```python
from build123d import *

# Parameters (mm, degrees)
CROQUIS1_R              = 1.75
SALIENTE_EXTRUIR1_DEPTH = 2
CROQUIS2_W              = 6
CROQUIS2_H              = 2
CORTAR_EXTRUIR1_DEPTH   = 1.2


with BuildPart() as part:
    # Croquis1 → Saliente-Extruir1 (new body)
    with BuildSketch(Plane(origin=(0, 0, 0), x_dir=(1, 0, 0), z_dir=(0, 1, 0))):
        with BuildLine():
            Line((-20.25, 0), (-20.25, 21))
            Line((-20.25, 21), (20.25, 21))
            Line((20.25, 21), (20.25, 0))
            Line((20.25, 0), (21.3, 0))
            Line((21.3, 0), (21.3, -3))
            Line((21.3, -3), (24.8, -3))
            Line((24.8, -3), (24.8, 0))
            Line((24.8, 0), (28.8, 0))
            Line((28.8, 0), (28.8, 18))
            ThreePointArc((28.8, 18), (27.335533906, 21.535533906), (23.8, 23))
            Line((23.8, 23), (-23.8, 23))
            ThreePointArc((-23.8, 23), (-27.335533906, 21.535533906), (-28.8, 18))
            Line((-28.8, 18), (-28.8, 0))
            Line((-28.8, 0), (-24.8, 0))
            Line((-24.8, 0), (-24.8, -3))
            Line((-24.8, -3), (-21.3, -3))
            Line((-21.3, -3), (-21.3, 0))
            Line((-21.3, 0), (-20.25, 0))
        make_face()
        with Locations(Location((-25, 5, 0), (0, 0, 270))):
            Circle(CROQUIS1_R, mode=Mode.SUBTRACT)
        with Locations(Location((25, 5, 0), (0, 0, 270))):
            Circle(CROQUIS1_R, mode=Mode.SUBTRACT)
        with Locations(Location((25, 16, 0), (0, 0, 270))):
            Circle(CROQUIS1_R, mode=Mode.SUBTRACT)
        with Locations(Location((-25, 16, 0), (0, 0, 270))):
            Circle(CROQUIS1_R, mode=Mode.SUBTRACT)
    extrude(amount=SALIENTE_EXTRUIR1_DEPTH)

    # Croquis2 → Cortar-Extruir1 (cut)
    with BuildSketch(Plane(origin=(0, 2, 0), x_dir=(1, 0, 0), z_dir=(0, 1, 0))):
        with Locations((-23.25, 10.5)):
            Rectangle(CROQUIS2_W, CROQUIS2_H)
        with Locations((23.25, 10.5)):
            Rectangle(CROQUIS2_W, CROQUIS2_H)
    extrude(amount=-CORTAR_EXTRUIR1_DEPTH, mode=Mode.SUBTRACT)


solid = part.part
```
CAD build for the part. Positions are in the model's coordinates, mm. A direction names the side the tool comes from. Coordinates: 2 decimals unless noted, no trailing zeros. Loops run counter-clockwise (first coordinate to the right, second up) from the corner with the lowest first, then second, coordinate; pieces in that order, holes last. Notation, with made-up numbers: (19.5, 71.25) - (27.5, 71.25) arc R27 cw to (27.5, 91.25) - close; hole circle Ø10 at (52, -11.5). An arc over 180 degrees is marked (long way). Return JSON: item names as keys, results as strings.
1. Probe L1, parallel to X at y = 0.8, z = -16; L2, parallel to X at y = 0.3, z = -9; L3, parallel to Z at x = -22.5, y = 1. List the from-to ranges inside material, lowest first. Write a range as from..to.
Result:
{"L1": "x = -28.8..-26.75, -23.25..-20.25, 20.25..23.25, 26.75..28.8", "L2": "x = -28.8..-20.25, 20.25..28.8", "L3": "z = -23..-11.5, -9.5..3"}
2. 3-axis set-ups, long thin cutter, end or side, ignore diameter. For faces 1 (the flat face through (24.8, 1, 2)), 2 (the flat face through (-20.25, 0.5, -10.4)), 3 (the flat face through (-23, 1, -11.5)): which of +Z, -Z, +X, -X, +Y, -Y reach the whole face in a straight line?
Result:
{"face 1": "+Z, +X, +Y, -Y", "face 2": "+Z, +Y, -Y", "face 3": "+Y"}
3. Mould opens along X. For faces 4 (the flat face through (0, 1, -21)), 5 (the flat face through (27, 1, 0)), 6 (the flat face through (-24.8, 1, 1)) say: released by +X, released by -X, zero draft, split by the parting line, or undercut.
Result:
{"face 4": "undercut", "face 5": "zero draft", "face 6": "released by -X"}
4. Drop flat-ended pins along their axis: pin 1 (1 mm diameter, centred on y = 1, z = 1.5, fed in from -X); pin 2 (0.6 mm diameter, centred on x = -2, y = 1, fed in from +Z); pin 3 (0.5 mm diameter, centred on x = 20.5, y = 0.5, fed in from +Z). Give the stop position or say it passes through.
Result:
{"pin 1": "stops at x = -24.8", "pin 2": "stops at z = -21", "pin 3": "stops at z = 0"}
5. Band-saw the part on D-D (x = 8). Give the cut face in (y, z).
Result:
{"outline": "(0, -23) - (2, -23) - (2, -21) - (0, -21) - close"}
6. Band-saw the part on A-A (z = -1.25). Give the cut face in (x, y).
Result:
{"outline": "(-28.8, 0) - (-20.25, 0) - (-20.25, 2) - (-28.8, 2) - close; (20.25, 0) - (28.8, 0) - (28.8, 2) - (20.25, 2) - close"}
7. Band-saw the part on C-C (z = -16). Give the cut face in (x, y), and give its area (3 significant figures).
Result:
{"outline": "(-28.8, 0) - (-26.75, 0) - (-26.75, 2) - (-28.8, 2) - close; (-23.25, 0) - (-20.25, 0) - (-20.25, 2) - (-23.25, 2) - close; (20.25, 0) - (23.25, 0) - (23.25, 2) - (20.25, 2) - close; (26.75, 0) - (28.8, 0) - (28.8, 2) - (26.75, 2) - close", "area": "20.2 mm2"}
8. Band-saw the part on B-B (y = 0.35). Give the cut face in (x, z), and give its area (3 significant figures).
Result:
{"outline": "(-28.8, -18) arc R5 ccw to (-23.8, -23) - (23.8, -23) arc R5 ccw to (28.8, -18) - (28.8, 0) - (24.8, 0) - (24.8, 3) - (21.3, 3) - (21.3, 0) - (20.25, 0) - (20.25, -21) - (-20.25, -21) - (-20.25, 0) - (-21.3, 0) - (-21.3, 3) - (-24.8, 3) - (-24.8, 0) - (-28.8, 0) - close; hole circle Ø3.5 at (-25, -16); hole circle Ø3.5 at (-25, -5); hole circle Ø3.5 at (25, -16); hole circle Ø3.5 at (25, -5)", "area": "446 mm2"}
